Autodesk Inventor part; units mm, degrees
ref_plane "YZ Plane" through (0, 0, 0) normal (1, 0, 0) x (0, 1, 0)
ref_plane "XZ Plane" through (0, 0, 0) normal (0, 1, 0) x (-1, 0, 0)
ref_plane "XY Plane" through (0, 0, 0) normal (0, 0, 1) x (1, 0, 0)
sketch "Sketch1" plane through (0, 0, 0) normal (0, 1, 0) x (-1, 0, 0)
  line L0 (-15.875, 28.575) -> (9.525, 28.575)
  line L1 (9.525, 28.575) -> (9.525, -9.525)
  line L2 (9.525, -9.525) -> (-15.875, -9.525)
  line L3 (-15.875, -9.525) -> (-15.875, 28.575)
  point P0 (0, 0)
  dimension "d0" = 38.1
  dimension "d1" = 25.4
  dimension "d2" = 9.525
  dimension "d3" = 9.525
extrude "Extrusion1" add sketch "Sketch1" along normal blind 3.175
sketch "Sketch4" plane through (-9.525, 0, -9.525) normal (-1, 0, 0) x (0, 0, 1)
  circle A0 centre (19.05, 27.0002) radius 14.2875
  line L0 (38.1, 0) -> (38.1, 3.175)
  line L1 (38.1, 3.175) -> (0, 3.175)
  line L2 (0, 0) -> (38.1, 0)
  line L3 (0, 0) -> (38.1, 0)
  line L4 (38.1, 0) -> (38.1, 50.8)
  line L5 (38.1, 50.8) -> (0, 50.8)
  line L6 (0, 50.8) -> (0, 0)
  point P0 (9.525, 0)
  dimension "d11" = 19.05
  dimension "d12" = 28.575
  dimension "d14" = 50.8
  dimension "d18" = 27.0002
  dimension "d19" = 38.1
extrude "Extrusion2" add sketch "Sketch4" against normal blind 3.175
fillet "Fillet1" radius 3.175 2 edges at (-7.9375, 50.8, 28.575) (-7.9375, 50.8, -9.525)
properties part number "ARM_011_BearingMount"
Geometry check sheet. Reference: the model listing, model coordinates, mm. A direction names the side the tool comes from. Round coordinates to 2 decimals unless told otherwise and drop trailing zeros. Loops run counter-clockwise (first coordinate to the right, second up) from the corner with the lowest first, then second, coordinate; pieces in that order, holes last. Notation, with made-up numbers: (25.5, -11) - (39.5, -11) arc R21 ccw to (39.5, 18) - close; hole circle Ø5 at (-27.5, -17). An arc over 180 degrees is marked (long way). Write item = value, one per line. Start each with the question number.
1. Section check A-A on z = 2.5. Enter the section's corners in (x, y) (3 decimals), then the cut area to 3 significant figures.
2. Section check B-B on y = 18. Enter the section's corners in (x, z) (3 decimals), then the cut area to 3 significant figures.
3. Thickness scan on line 1 (X direction, y = 39.5, z = 19.5) (3 decimals); line 2 (Y direction, x = 6, z = 13.5) (3 decimals); line 3 (Z direction, x = -7.5, y = 22.5) (3 decimals). Record the ranges inside material, lowest first.
4. Depth check by flat-ended pin: pin 1 (8 mm diameter, centred on x = 4.5, z = 13.5, fed in from +Y) (3 decimals); pin 2 (2 mm diameter, centred on y = 27.5, z = -4, fed in from -X) (3 decimals); pin 3 (11.5 mm diameter, centred on y = 36.5, z = 17.5, fed in from +X). Enter the tip coordinate at first touch or a pass-through.
5. Mould release check, pull along Z, two halves, no side actions. Record for faces 3 (the face through (-7, 17, -9.525)), 4 (the face through (-8, 50.8, 10)), 5 (the face through (-7.96, 31.292, 23.153)): released by +Z, released by -Z, zero draft, split by the parting line, or undercut.
6. Set-up check for faces 1 (the face through (-6.35, 11, 9)), 2 (the face through (3, 0, 10)): record each of +Z, -Z, +X, -X, +Y, -Y from which the full face is reachable in a straight line by a thin tool's end or side.
7. Section check C-C on x = -0.5. Enter the section's corners in (y, z) (3 decimals).
Working result:
q1.outline = (-9.525, 0) - (15.875, 0) - (15.875, 3.175) - (-6.35, 3.175) - (-6.35, 14.559) - (-9.525, 14.559) - close; (-9.525, 39.441) - (-6.35, 39.441) - (-6.35, 50.8) - (-9.525, 50.8) - close
q1.area = 153 mm^2
q2.outline = (-9.525, -9.525) - (-6.35, -9.525) - (-6.35, -1.571) - (-9.525, -1.571) - close; (-9.525, 20.621) - (-6.35, 20.621) - (-6.35, 28.575) - (-9.525, 28.575) - close
q2.area = 50.5 mm^2
q3.line_1 = -9.525 to -6.35
q3.line_2 = 0 to 3.175
q3.line_3 = -9.525 to -4.035, 23.085 to 28.575
q4.pin_1 = 3.175
q4.pin_2 = -9.525
q4.pin_3 = -6.35
q5.face_3 = released by -Z
q5.face_4 = zero draft
q5.face_5 = undercut
q6.face_1 = +Z, -Z, +X, +Y
q6.face_2 = +Z, -Z, +X, -X, -Y
q7.outline = (0, -9.525) - (3.175, -9.525) - (3.175, 28.575) - (0, 28.575) - close
